Geometry check sheet. Reference: drawing and pictorial views, mm from the part's lowest x, y, z. A direction names the side the tool comes from. Coordinates: 2 decimals unless noted, no trailing zeros. Write each loop counter-clockwise with the first axis right and the second up, starting at its lowest first coordinate (ties: lowest second). Pieces come first, ordered by that corner, then holes. Notation, with made-up numbers: (48.5, 49) - (64.5, 49) arc R16 ccw to (64.5, 73) - close; hole circle Ø3 at (-4, 1.5). An arc over 180 degrees is marked (long way). Use one line per item in the form item = value. Start each with the question number.
(1) Gauge pin test, flat ends, axial feed: pin 1 Ø2 at (y, z) = (15.5, 25.5) entering from +X; pin 2 Ø3 at (y, z) = (5, 54) entering from +X; pin 3 Ø5 at (x, y) = (7, 5.5) entering from +Z. Record the tip position at first contact, or that the pin passes through.
(2) Tool access check on the marked faces 1 and 2. Record the directions out of +Z, -Z, +X, -X, +Y, -Y that give a thin tool (end or side, any length) a straight path to the whole face; none if there is none.
(3) Material ranges on line 1 (Z direction, x = 25, y = 12.5); line 2 (Z direction, x = 21.25, y = 23.5); line 3 (X direction, y = 8.5, z = 8), recorded low to high. Write a range as [from, to].
(4) Sectioned sample at D-D (x = 5). Record the cut outline in (y, z).
(5) Sectioned sample at C-C (z = 21). Record the cut outline in (x, y).
(6) Sectioned sample at B-B (x = 13.5). Record the cut outline in (y, z), and give its area (3 significant figures).
(7) Mould release check, pull along Z, two halves, no side actions. Record for the marked faces 3, 4 and 5: released by +Z, released by -Z, zero draft, split by the parting line, or undercut.
(8) Sectioned sample at A-A (y = 13.5). Record the cut outline in (x, z), and give its area (3 significant figures).
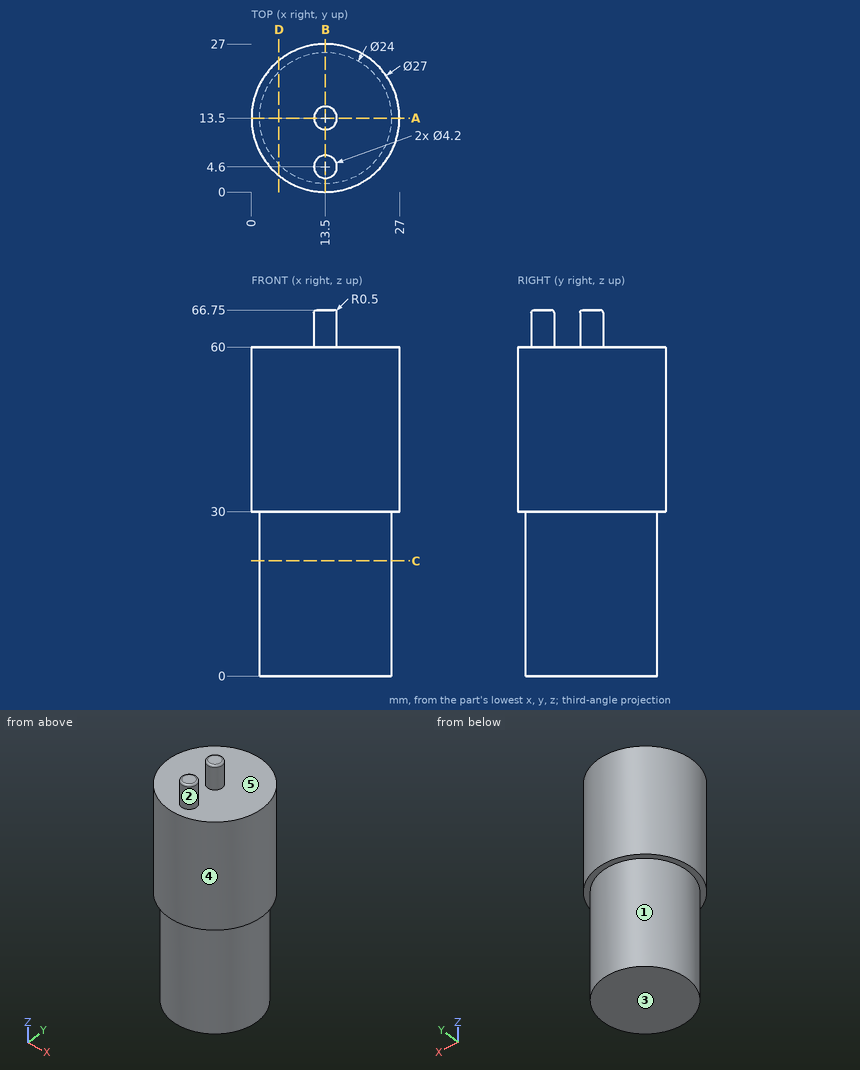
Answers below:
q1.pin_1 = 25.46
q1.pin_2 = 25.04
q1.pin_3 = 60
q2.face_1 = -Z
q2.face_2 = +Z
q3.line_1 = [0, 60]
q3.line_2 = [30, 60]
q3.line_3 = [2.59, 24.41]
q4.outline = (3.01, 30) - (5.03, 30) - (5.03, 0) - (21.97, 0) - (21.97, 30) - (23.99, 30) - (23.99, 60) - (3.01, 60) - close
q5.outline = circle Ø24 at (13.5, 13.5)
q6.outline = (0, 30) - (1.5, 30) - (1.5, 0) - (25.5, 0) - (25.5, 30) - (27, 30) - (27, 60) - (15.6, 60) - (15.6, 66.25) arc R0.5 ccw to (15.1, 66.75) - (11.9, 66.75) arc R0.5 ccw to (11.4, 66.25) - (11.4, 60) - (6.7, 60) - (6.7, 66.25) arc R0.5 ccw to (6.2, 66.75) - (3, 66.75) arc R0.5 ccw to (2.5, 66.25) - (2.5, 60) - (0, 60) - close
q6.area = 1,590 mm2
q7.face_3 = released by -Z
q7.face_4 = zero draft
q7.face_5 = released by +Z
q8.outline = (0, 30) - (1.5, 30) - (1.5, 0) - (25.5, 0) - (25.5, 30) - (27, 30) - (27, 60) - (15.6, 60) - (15.6, 66.25) arc R0.5 ccw to (15.1, 66.75) - (11.9, 66.75) arc R0.5 ccw to (11.4, 66.25) - (11.4, 60) - (0, 60) - close
q8.area = 1,560 mm2
